from build123d import *

# Parameters (mm, degrees)
SKETCH1_W               = 60
SKETCH1_H               = 35
BOSS_EXTRUDE1_DEPTH     = 10
SKETCH2_W               = 22
SKETCH2_H               = 10
CUT_EXTRUDE1_DEPTH      = 19
SKETCH3_W               = 22
SKETCH3_H               = 10
CUT_EXTRUDE2_DEPTH      = 29
SKETCH5_R               = 1.45
CUT_EXTRUDE4_DEPTH      = 71.178344238
FILLET1_R               = 3
FILLET2_R               = 3
SKETCH7_W               = 12
SKETCH7_H               = 10
BOSS_EXTRUDE2_DEPTH     = 3
CUT_EXTRUDE5_DEPTH      = 3
CUT_EXTRUDE5_DEPTH_BACK = 15
SKETCH6_R               = 1.45
FILLET3_R               = 4


with BuildPart() as part:
    # Sketch1 → Boss-Extrude1 (new body)
    with BuildSketch(Plane(origin=(0, 0, 0), x_dir=(1, 0, 0), z_dir=(0, 1, 0))):
        with Locations((30, -17.5)):
            Rectangle(SKETCH1_W, SKETCH1_H)
    extrude(amount=BOSS_EXTRUDE1_DEPTH)

    # Sketch2 → Cut-Extrude1 (cut)
    with BuildSketch(Plane(origin=(60, 0, 0), x_dir=(0, 0, -1), z_dir=(1, 0, 0))):
        with Locations((-17.5, 5)):
            Rectangle(SKETCH2_W, SKETCH2_H)
    extrude(amount=-CUT_EXTRUDE1_DEPTH, mode=Mode.SUBTRACT)

    # Sketch3 → Cut-Extrude2 (cut)
    with BuildSketch(Plane.ZY):
        with Locations((17.5, 5)):
            Rectangle(SKETCH3_W, SKETCH3_H)
    extrude(amount=-CUT_EXTRUDE2_DEPTH, mode=Mode.SUBTRACT)

    # Sketch5 → Cut-Extrude4 (cut, through all)
    with BuildSketch(Plane.XY.offset(35)):
        with Locations((5, 5)):
            Circle(SKETCH5_R)
        with Locations((55, 5)):
            Circle(SKETCH5_R)
    extrude(amount=-CUT_EXTRUDE4_DEPTH, mode=Mode.SUBTRACT)

    # Fillet1
    fillet1_edges = [part.edges().sort_by_distance(p)[0] for p in [
        (60, 10, 31.75),
        (60, 0, 3.25),
        (60, 10, 3.25),
        (0, 0, 31.75),
        (0, 10, 31.75),
        (0, 10, 3.25),
        (60, 0, 31.75),
        (0, 0, 3.25),
    ]]
    fillet(fillet1_edges, radius=FILLET1_R)

    # Fillet2
    fillet2_edges = [part.edges().sort_by_distance(p)[0] for p in [
        (41, 5, 28.5),
        (41, 5, 6.5),
        (29, 5, 6.5),
        (29, 5, 28.5),
    ]]
    fillet(fillet2_edges, radius=FILLET2_R)

    # Sketch7 → Boss-Extrude2 (add)
    with BuildSketch(Plane.XY.offset(35)):
        with Locations((35, 5)):
            Rectangle(SKETCH7_W, SKETCH7_H)
    extrude(amount=BOSS_EXTRUDE2_DEPTH)

    # Sketch6 → Cut-Extrude5 (cut, two sides: drawn at the far end of the back side and taken through both)
    with BuildSketch(Plane.XY.offset(35).offset(-CUT_EXTRUDE5_DEPTH_BACK)):
        with Locations((34.5, 5)):
            Circle(SKETCH6_R)
    extrude(amount=CUT_EXTRUDE5_DEPTH + CUT_EXTRUDE5_DEPTH_BACK, mode=Mode.SUBTRACT)

    # Fillet3
    # the kernel refuses this fillet: 4 mm, written as the material it adds along each edge
    with BuildSketch(Plane(origin=(41, 10, 35), x_dir=(0, 0, 1), z_dir=(0, -1, 0))) as fillet3_piece_1:
        with BuildLine():
            CenterArc((4, -3.872983346), FILLET3_R, 104.477512186, 75.522487814)
            Line((0, -3.872983346), (-0.08, -3.872983346))
            Line((-0.08, -3.872983346), (-0.08, 0))
            Line((-0.08, 0), (0, 0.08))
            ThreePointArc((0, 0.08), (1.5, 0.08), (2.98, 0.077459667))
            Line((2.98, 0.077459667), (3, 0))
        make_face()
    extrude(amount=10)
    with BuildSketch(Plane(origin=(29, 0, 35), x_dir=(-1, 0, 0), z_dir=(0, 1, 0))) as fillet3_piece_2:
        with BuildLine():
            CenterArc((3.872983346, 4), FILLET3_R, 194.477512186, 75.522487814)
            Line((0, 3), (-0.077459667, 2.98))
            ThreePointArc((-0.077459667, 2.98), (-0.08, 1.5), (-0.08, 0))
            Line((-0.08, 0), (0, -0.08))
            Line((0, -0.08), (3.872983346, -0.08))
            Line((3.872983346, -0.08), (3.872983346, 0))
        make_face()
    extrude(amount=10)


solid = part.part
Verification items for the finished model (mm, model axes). A direction names the side the tool comes from. Give positions to 0.01 mm unless a question says otherwise; leave off trailing zeros. Loops run counter-clockwise (first coordinate to the right, second up) from the corner with the lowest first, then second, coordinate; pieces in that order, holes last. Notation, with made-up numbers: (-31, 82.25) - (-21, 82.25) arc R29 ccw to (-21, 110.25) - close; hole circle Ø11 at (10, 40.25). An arc over 180 degrees is marked (long way). Write item = value, one per line. Start each with the question number.
Q1. Mould release check, pull along Z, two halves, no side actions. Record for faces 4 (the face through (52, 5, 6.5)), 5 (the face through (28.14, 5.07, 7.4)), 6 (the face through (30, 10, 19)), 7 (the face through (12, 5, 35)): released by +Z, released by -Z, zero draft, split by the parting line, or undercut.
Q2. Cross-section at C-C, the plane y = 5. State how many separate pieces and enclosed holes the cut face has, and give its area (3 significant figures).
Q3. Tool access check on faces 1 (the face through (52, 5, 28.5)), 2 (the face through (52, 5, 35)), 3 (the face through (30, 0, 19)). Record the directions out of +Z, -Z, +X, -X, +Y, -Y that give a thin tool (end or side, any length) a straight path to the whole face; none if there is none.
Q4. Thickness scan on line 1 (Y direction, x = 55, z = 33); line 2 (Z direction, x = 54, y = 7.5); line 3 (Z direction, x = 27.5, y = 2). Record the ranges inside material, lowest first.
Q5. Depth check by flat-ended pin: P1, Ø5, axis at y = 2, z = 22, coming from the +X side; P2, Ø3, axis at x = 51.5, y = 5, coming from the +Z side; P3, Ø1.7, axis at x = 34.5, y = 5, coming from the +Z side. Enter the tip coordinate at first touch or a pass-through.
Q6. Cross-section at D-D, the plane x = 34.5. Enter the section's corners in (y, z).
Q7. Cross-section at B-B, the plane z = 33. Enter the section's corners in (x, y).
Q8. Cross-section at A-A, the plane x = 55. Enter the section's corners in (y, z).
Answer key:
q1.face_4 = undercut
q1.face_5 = undercut
q1.face_6 = zero draft
q1.face_7 = released by +Z
q2.separate_pieces = 5
q2.enclosed_holes = 0
q2.area = 966 mm^2
q3.face_1 = +X, +Y, -Y
q3.face_2 = +Z, +X, +Y, -Y
q3.face_3 = +Z, -Z, +X, -X, -Y
q4.line_1 = 0 to 3.55, 6.45 to 10
q4.line_2 = 0 to 6.5, 28.5 to 35
q4.line_3 = 0 to 6.9, 28.1 to 35.78
q5.P1 = 41
q5.P2 = 35
q5.P3 = 20
q6.outline = (0, 0) - (10, 0) - (10, 38) - (6.45, 38) - (6.45, 20) - (3.55, 20) - (3.55, 38) - (0, 38) - close
q7.outline = (0, 3) arc R3 ccw to (3, 0) - (57, 0) arc R3 ccw to (60, 3) - (60, 7) arc R3 ccw to (57, 10) - (3, 10) arc R3 ccw to (0, 7) - close; hole circle Ø2.9 at (5, 5); hole circle Ø2.9 at (34.5, 5); hole circle Ø2.9 at (55, 5)
q8.outline = (0, 0) - (3.55, 0) - (3.55, 6.5) - (0, 6.5) - close; (0, 28.5) - (3.55, 28.5) - (3.55, 35) - (0, 35) - close; (6.45, 0) - (10, 0) - (10, 6.5) - (6.45, 6.5) - close; (6.45, 28.5) - (10, 28.5) - (10, 35) - (6.45, 35) - close
